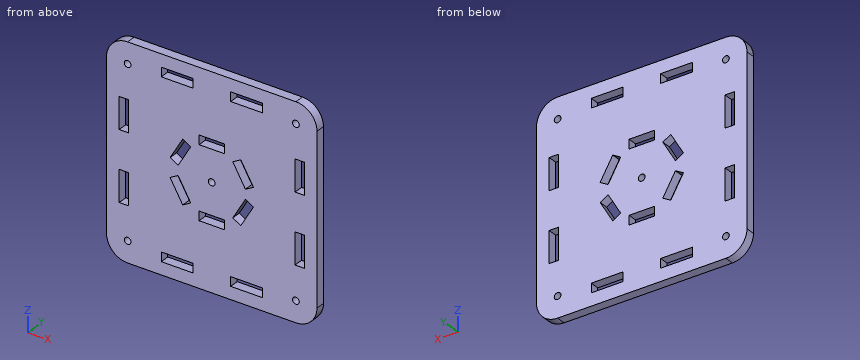
```python
from build123d import *

# Parameters (mm, degrees)
SKETCH_1_W          = 100
SKETCH_1_H          = 100
SKETCH_1_R          = 1.6
EXTRUDE_1_DEPTH     = 4.4
FILLET_1_R          = 10
CUT_EXTRUDE_1_REACH = 6.4
SKETCH_2_R          = 1.6
SKETCH_2_W          = 15
SKETCH_2_H          = 4.4
SKETCH_2_W_2        = 4.4
SKETCH_2_H_2        = 15
SKETCH_3_W          = 12
SKETCH_3_H          = 4.4
CUT_EXTRUDE_2_DEPTH = 5.4


with BuildPart() as part:
    # 草图1 → 凸台-拉伸1 (new body)
    with BuildSketch(Plane(origin=(0, 0, 0), x_dir=(1, 0, 0), z_dir=(0, 1, 0))):
        Rectangle(SKETCH_1_W, SKETCH_1_H)
        Circle(SKETCH_1_R, mode=Mode.SUBTRACT)
    extrude(amount=EXTRUDE_1_DEPTH)

    # 圆角1
    fillet_1_edges = [part.edges().sort_by_distance(p)[0] for p in [
        (50, 2.2, 50),
        (-50, 2.2, 50),
        (-50, 2.2, -50),
        (50, 2.2, -50),
    ]]
    fillet(fillet_1_edges, radius=FILLET_1_R)

    # 草图2 → 切除-拉伸1 (cut, up to next)
    with BuildSketch(Plane(origin=(0, 4.4, 0), x_dir=(1, 0, 0), z_dir=(0, 1, 0)), mode=Mode.PRIVATE) as cut_extrude_1_sk1:
        with Locations((40, 40)):
            Circle(SKETCH_2_R)
    cut_extrude_1_tool1 = extrude(cut_extrude_1_sk1.sketch, amount=-CUT_EXTRUDE_1_REACH, mode=Mode.PRIVATE) & part.part
    add(cut_extrude_1_tool1.solids().sort_by_distance((40, 4.4, -40))[0], mode=Mode.SUBTRACT)
    # 草图2 → 切除-拉伸1 (cut, up to next)
    with BuildSketch(Plane(origin=(0, 4.4, 0), x_dir=(1, 0, 0), z_dir=(0, 1, 0)), mode=Mode.PRIVATE) as cut_extrude_1_sk2:
        with Locations((40, -40)):
            Circle(SKETCH_2_R)
    cut_extrude_1_tool2 = extrude(cut_extrude_1_sk2.sketch, amount=-CUT_EXTRUDE_1_REACH, mode=Mode.PRIVATE) & part.part
    add(cut_extrude_1_tool2.solids().sort_by_distance((40, 4.4, 40))[0], mode=Mode.SUBTRACT)
    # 草图2 → 切除-拉伸1 (cut, up to next)
    with BuildSketch(Plane(origin=(0, 4.4, 0), x_dir=(1, 0, 0), z_dir=(0, 1, 0)), mode=Mode.PRIVATE) as cut_extrude_1_sk3:
        with Locations((-40, -40)):
            Circle(SKETCH_2_R)
    cut_extrude_1_tool3 = extrude(cut_extrude_1_sk3.sketch, amount=-CUT_EXTRUDE_1_REACH, mode=Mode.PRIVATE) & part.part
    add(cut_extrude_1_tool3.solids().sort_by_distance((-40, 4.4, 40))[0], mode=Mode.SUBTRACT)
    # 草图2 → 切除-拉伸1 (cut, up to next)
    with BuildSketch(Plane(origin=(0, 4.4, 0), x_dir=(1, 0, 0), z_dir=(0, 1, 0)), mode=Mode.PRIVATE) as cut_extrude_1_sk4:
        with Locations((-40, 40)):
            Circle(SKETCH_2_R)
    cut_extrude_1_tool4 = extrude(cut_extrude_1_sk4.sketch, amount=-CUT_EXTRUDE_1_REACH, mode=Mode.PRIVATE) & part.part
    add(cut_extrude_1_tool4.solids().sort_by_distance((-40, 4.4, -40))[0], mode=Mode.SUBTRACT)
    # 草图2 → 切除-拉伸1 (cut, up to next)
    with BuildSketch(Plane(origin=(0, 4.4, 0), x_dir=(1, 0, 0), z_dir=(0, 1, 0)), mode=Mode.PRIVATE) as cut_extrude_1_sk5:
        with Locations((-16.5, 41.8)):
            Rectangle(SKETCH_2_W, SKETCH_2_H)
    cut_extrude_1_tool5 = extrude(cut_extrude_1_sk5.sketch, amount=-CUT_EXTRUDE_1_REACH, mode=Mode.PRIVATE) & part.part
    add(cut_extrude_1_tool5.solids().sort_by_distance((-16.5, 4.4, -41.8))[0], mode=Mode.SUBTRACT)
    # 草图2 → 切除-拉伸1 (cut, up to next)
    with BuildSketch(Plane(origin=(0, 4.4, 0), x_dir=(1, 0, 0), z_dir=(0, 1, 0)), mode=Mode.PRIVATE) as cut_extrude_1_sk6:
        with Locations((16.5, 41.8)):
            Rectangle(SKETCH_2_W, SKETCH_2_H)
    cut_extrude_1_tool6 = extrude(cut_extrude_1_sk6.sketch, amount=-CUT_EXTRUDE_1_REACH, mode=Mode.PRIVATE) & part.part
    add(cut_extrude_1_tool6.solids().sort_by_distance((16.5, 4.4, -41.8))[0], mode=Mode.SUBTRACT)
    # 草图2 → 切除-拉伸1 (cut, up to next)
    with BuildSketch(Plane(origin=(0, 4.4, 0), x_dir=(1, 0, 0), z_dir=(0, 1, 0)), mode=Mode.PRIVATE) as cut_extrude_1_sk7:
        with Locations((41.8, -16.5)):
            Rectangle(SKETCH_2_W_2, SKETCH_2_H_2)
    cut_extrude_1_tool7 = extrude(cut_extrude_1_sk7.sketch, amount=-CUT_EXTRUDE_1_REACH, mode=Mode.PRIVATE) & part.part
    add(cut_extrude_1_tool7.solids().sort_by_distance((41.8, 4.4, 16.5))[0], mode=Mode.SUBTRACT)
    # 草图2 → 切除-拉伸1 (cut, up to next)
    with BuildSketch(Plane(origin=(0, 4.4, 0), x_dir=(1, 0, 0), z_dir=(0, 1, 0)), mode=Mode.PRIVATE) as cut_extrude_1_sk8:
        with Locations((41.8, 16.5)):
            Rectangle(SKETCH_2_W_2, SKETCH_2_H_2)
    cut_extrude_1_tool8 = extrude(cut_extrude_1_sk8.sketch, amount=-CUT_EXTRUDE_1_REACH, mode=Mode.PRIVATE) & part.part
    add(cut_extrude_1_tool8.solids().sort_by_distance((41.8, 4.4, -16.5))[0], mode=Mode.SUBTRACT)
    # 草图2 → 切除-拉伸1 (cut, up to next)
    with BuildSketch(Plane(origin=(0, 4.4, 0), x_dir=(1, 0, 0), z_dir=(0, 1, 0)), mode=Mode.PRIVATE) as cut_extrude_1_sk9:
        with Locations((-16.5, -41.8)):
            Rectangle(SKETCH_2_W, SKETCH_2_H)
    cut_extrude_1_tool9 = extrude(cut_extrude_1_sk9.sketch, amount=-CUT_EXTRUDE_1_REACH, mode=Mode.PRIVATE) & part.part
    add(cut_extrude_1_tool9.solids().sort_by_distance((-16.5, 4.4, 41.8))[0], mode=Mode.SUBTRACT)
    # 草图2 → 切除-拉伸1 (cut, up to next)
    with BuildSketch(Plane(origin=(0, 4.4, 0), x_dir=(1, 0, 0), z_dir=(0, 1, 0)), mode=Mode.PRIVATE) as cut_extrude_1_sk10:
        with Locations((16.5, -41.8)):
            Rectangle(SKETCH_2_W, SKETCH_2_H)
    cut_extrude_1_tool10 = extrude(cut_extrude_1_sk10.sketch, amount=-CUT_EXTRUDE_1_REACH, mode=Mode.PRIVATE) & part.part
    add(cut_extrude_1_tool10.solids().sort_by_distance((16.5, 4.4, 41.8))[0], mode=Mode.SUBTRACT)
    # 草图2 → 切除-拉伸1 (cut, up to next)
    with BuildSketch(Plane(origin=(0, 4.4, 0), x_dir=(1, 0, 0), z_dir=(0, 1, 0)), mode=Mode.PRIVATE) as cut_extrude_1_sk11:
        with Locations((-41.8, 16.5)):
            Rectangle(SKETCH_2_W_2, SKETCH_2_H_2)
    cut_extrude_1_tool11 = extrude(cut_extrude_1_sk11.sketch, amount=-CUT_EXTRUDE_1_REACH, mode=Mode.PRIVATE) & part.part
    add(cut_extrude_1_tool11.solids().sort_by_distance((-41.8, 4.4, -16.5))[0], mode=Mode.SUBTRACT)
    # 草图2 → 切除-拉伸1 (cut, up to next)
    with BuildSketch(Plane(origin=(0, 4.4, 0), x_dir=(1, 0, 0), z_dir=(0, 1, 0)), mode=Mode.PRIVATE) as cut_extrude_1_sk12:
        with Locations((-41.8, -16.5)):
            Rectangle(SKETCH_2_W_2, SKETCH_2_H_2)
    cut_extrude_1_tool12 = extrude(cut_extrude_1_sk12.sketch, amount=-CUT_EXTRUDE_1_REACH, mode=Mode.PRIVATE) & part.part
    add(cut_extrude_1_tool12.solids().sort_by_distance((-41.8, 4.4, 16.5))[0], mode=Mode.SUBTRACT)

    # 草图3 → 切除-拉伸2 (cut, through all)
    with BuildSketch(Plane(origin=(0, 4.4, 0), x_dir=(1, 0, 0), z_dir=(0, 1, 0))):
        with Locations((0, 17.2)):
            Rectangle(SKETCH_3_W, SKETCH_3_H)
        Polygon((13.800892833, 14.896152423), (9.990381057, 12.696152423), (15.990381057, 2.303847577), (19.800892833, 4.503847577), align=None)
        Polygon((19.800892833, -4.503847577), (15.990381057, -2.303847577), (9.990381057, -12.696152423), (13.800892833, -14.896152423), align=None)
        with Locations((0, -17.2)):
            Rectangle(SKETCH_3_W, SKETCH_3_H)
        Polygon((-13.800892833, -14.896152423), (-9.990381057, -12.696152423), (-15.990381057, -2.303847577), (-19.800892833, -4.503847577), align=None)
        Polygon((-19.800892833, 4.503847577), (-15.990381057, 2.303847577), (-9.990381057, 12.696152423), (-13.800892833, 14.896152423), align=None)
    extrude(amount=-CUT_EXTRUDE_2_DEPTH, mode=Mode.SUBTRACT)


solid = part.part
```
For this review, take the finished solid that the model builds, in its own axes (mm). Coordinates: 2 decimals unless noted, no trailing zeros. Order: outer loops, then holes, each group sorted by start corner. A loop starts at its lowest first (then second) coordinate and runs counter-clockwise, first axis right, second up. Notation, with made-up numbers: (80, 55.5) -> (114, 55.5) arc R34 ccw to (114, 88.5) -> close; hole circle Ø4 at (-36, 70.25). An arc over 180 degrees is marked (long way). Use CSV: the item, a comma, the result in double quotes. Start each with the question number.
Item 1: We need section B-B, the plane z = 17.5. Give the boundary of the cut face in (x, y).
Item 2: We need section A-A, the plane x = 0. Give the boundary of the cut face in (y, z), then the cut area to 3 significant figures.
Item 3: Wall thickness on probe 1 along Z at (x, y) = (-40, 1.8); probe 2 along Z at (x, y) = (13, 4.2): over which ranges is each line inside the solid? List them lowest first.
Item 4: We need section C-C, the plane z = 0. Give the boundary of the cut face in (x, y).
Item 5: Insertion check: pin 1 (2 mm diameter, centred on x = 41.5, y = 2.5, fed in from -Z). The pin has a flat end and moves straight along its axis. Give the tip position at first contact, or say it passes through.
Item 6: We need section D-D, the plane y = 1.05. Give the number of separate pieces and of enclosed holes in the cut face, then the cut area to 3 significant figures.
Derived:
1,outline,"(-50, 0) -> (-44, 0) -> (-44, 4.4) -> (-50, 4.4) -> close; (-39.6, 0) -> (-6, 0) -> (-6, 4.4) -> (-39.6, 4.4) -> close; (6, 0) -> (39.6, 0) -> (39.6, 4.4) -> (6, 4.4) -> close; (44, 0) -> (50, 0) -> (50, 4.4) -> (44, 4.4) -> close"
2,outline,"(0, -50) -> (4.4, -50) -> (4.4, -19.4) -> (0, -19.4) -> close; (0, -15) -> (4.4, -15) -> (4.4, -1.6) -> (0, -1.6) -> close; (0, 1.6) -> (4.4, 1.6) -> (4.4, 15) -> (0, 15) -> close; (0, 19.4) -> (4.4, 19.4) -> (4.4, 50) -> (0, 50) -> close"
2,area,"387 mm^2"
3,probe 1,"z = -50 to -41.6, -38.4 to -24, -9 to 9, 24 to 38.4, 41.6 to 50"
3,probe 2,"z = -50 to -44, -39.6 to -14.43, -7.48 to 7.48, 14.43 to 39.6, 44 to 50"
4,outline,"(-50, 0) -> (-1.6, 0) -> (-1.6, 4.4) -> (-50, 4.4) -> close; (1.6, 0) -> (50, 0) -> (50, 4.4) -> (1.6, 4.4) -> close"
5,pin 1,"stops at z = -49.99"
6,separate pieces,"1"
6,enclosed holes,"19"
6,area,"9,030 mm^2"
